Geometry: final body of the model. Coordinates: model frame, mm. Give positions to 0.01 mm unless a question says otherwise; leave off trailing zeros. Write each loop counter-clockwise with the first axis right and the second up, starting at its lowest first coordinate (ties: lowest second). Pieces come first, ordered by that corner, then holes.
Q1. Line query: L1, parallel to X at y = -1.5, z = 0.1; L2, parallel to Y at x = 2.75, z = 0.1; L3, parallel to Y at x = -2, z = 0.15. Output: solid intervals per line, ascending.
Q2. Cut plane D-D on x = 2.5. Return the cut outline in (y, z), plus the area to 3 significant figures.
Q3. Cut plane C-C on y = 2. Return the cut outline in (x, z), plus the area to 3 significant figures.
Q4. Draft query along Y for faces 1 (the face through (1, 0, 0)), 2 (the face through (2.57, -0.62, 0.15)), 3 (the face through (-3.32, 3.04, 0.15)). Return one class per face: pulls with the +Y half, pulls with the -Y half, needs draft (parallel to the pull), parting line crosses it, or undercut.
Q5. Cut plane B-B on y = 0. Return the cut outline in (x, z), plus the area to 3 significant figures.
Q6. Cut plane A-A on x = 0. Return the cut outline in (y, z), plus the area to 3 significant figures.
```python
from build123d import *

# Parameters (mm, degrees)
SKETCH1_R           = 4.5
SKETCH1_R_2         = 0.75
BOSS_EXTRUDE1_DEPTH = 0.3
SKETCH2_R           = 0.25
CUT_EXTRUDE1_DEPTH  = 0.3
SKETCH3_W           = 1.6
SKETCH3_H           = 3
CUT_EXTRUDE2_DEPTH  = 0.3
FILLET1_R           = 0.2
SKETCH4_R           = 0.15
CUT_EXTRUDE3_DEPTH  = 0.3
CIRPATTERN1_COUNT   = 3
SKETCH5_R           = 0.15
CUT_EXTRUDE4_DEPTH  = 0.3
CIRPATTERN3_COUNT   = 3
SKETCH6_R           = 0.15
CUT_EXTRUDE5_DEPTH  = 0.3
CIRPATTERN4_COUNT   = 3
SKETCH7_R           = 0.15
CUT_EXTRUDE8_DEPTH  = 0.3


with BuildPart() as part:
    # Sketch1 → Boss-Extrude1 (new body)
    with BuildSketch(Plane.XY):
        Circle(SKETCH1_R)
        with Locations((0, 2.5)):
            Circle(SKETCH1_R_2, mode=Mode.SUBTRACT)
        with Locations((2.165063509, -1.25)):
            Circle(SKETCH1_R_2, mode=Mode.SUBTRACT)
        with Locations((-2.165063509, -1.25)):
            Circle(SKETCH1_R_2, mode=Mode.SUBTRACT)
    extrude(amount=BOSS_EXTRUDE1_DEPTH)

    # Sketch2 → Cut-Extrude1 (cut)
    with BuildSketch(Plane.XY.offset(0.3)):
        with Locations((0, -4)):
            Circle(SKETCH2_R)
        with Locations((-3.464101615, -2)):
            Circle(SKETCH2_R)
        with Locations((-3.464101615, 2)):
            Circle(SKETCH2_R)
        with Locations((0, 4)):
            Circle(SKETCH2_R)
        with Locations((3.464101615, 2)):
            Circle(SKETCH2_R)
        with Locations((3.464101615, -2)):
            Circle(SKETCH2_R)
    extrude(amount=-CUT_EXTRUDE1_DEPTH, mode=Mode.SUBTRACT)

    # Sketch3 → Cut-Extrude2 (cut)
    with BuildSketch(Plane.XY.offset(0.3)):
        with Locations((0, -1)):
            Rectangle(SKETCH3_W, SKETCH3_H)
    extrude(amount=-CUT_EXTRUDE2_DEPTH, mode=Mode.SUBTRACT)

    # Fillet1
    fillet1_edges = [part.edges().sort_by_distance(p)[0] for p in [
        (-0.8, 0.5, 0.15),
        (0.8, 0.5, 0.15),
        (0.8, -2.5, 0.15),
        (-0.8, -2.5, 0.15),
    ]]
    fillet(fillet1_edges, radius=FILLET1_R)

    # Sketch4 → Cut-Extrude3 (cut)
    with BuildSketch(Plane.XY.offset(0.3)):
        with Locations((0, 3.5)):
            Circle(SKETCH4_R)
    cut_extrude3 = extrude(amount=-CUT_EXTRUDE3_DEPTH, mode=Mode.SUBTRACT)

    # CirPattern1: Cut-Extrude3 ×3 about axis
    cirpattern1_axis = Axis((0, 2.5, 0), (0, 0, 1))
    for i in range(1, CIRPATTERN1_COUNT):
        add(cut_extrude3.rotate(cirpattern1_axis, i * 360 / CIRPATTERN1_COUNT), mode=Mode.SUBTRACT)

    # Sketch5 → Cut-Extrude4 (cut)
    with BuildSketch(Plane.XY.offset(0.3)):
        with Locations((3.165063509, -1.25)):
            Circle(SKETCH5_R)
    cut_extrude4 = extrude(amount=-CUT_EXTRUDE4_DEPTH, mode=Mode.SUBTRACT)

    # CirPattern3: Cut-Extrude4 ×3 about axis
    cirpattern3_axis = Axis((2.165063509, -1.25, 0), (0, 0, 1))
    for i in range(1, CIRPATTERN3_COUNT):
        add(cut_extrude4.rotate(cirpattern3_axis, i * 360 / CIRPATTERN3_COUNT), mode=Mode.SUBTRACT)

    # Sketch6 → Cut-Extrude5 (cut)
    with BuildSketch(Plane.XY.offset(0.3)):
        with Locations((-3.165063509, -1.25)):
            Circle(SKETCH6_R)
    cut_extrude5 = extrude(amount=-CUT_EXTRUDE5_DEPTH, mode=Mode.SUBTRACT)

    # CirPattern4: Cut-Extrude5 ×3 about axis
    cirpattern4_axis = Axis((-2.165063509, -1.25, 0), (0, 0, 1))
    for i in range(1, CIRPATTERN4_COUNT):
        add(cut_extrude5.rotate(cirpattern4_axis, i * 360 / CIRPATTERN4_COUNT), mode=Mode.SUBTRACT)

    # Sketch7 → Cut-Extrude8 (cut)
    with BuildSketch(Plane.XY.offset(0.3)):
        with Locations((0.4, -3)):
            Circle(SKETCH7_R)
        with Locations((-0.4, -3)):
            Circle(SKETCH7_R)
        with Locations((0.4, 1)):
            Circle(SKETCH7_R)
        with Locations((-0.4, 1)):
            Circle(SKETCH7_R)
    extrude(amount=-CUT_EXTRUDE8_DEPTH, mode=Mode.SUBTRACT)


solid = part.part
```
Data:
1. L1: x = -4.24 to -2.87, -1.46 to -0.8, 0.8 to 1.46, 2.87 to 4.24
1. L2: y = -3.56 to -1.72, -0.78 to 3.56
1. L3: y = -4.03 to -1.98, -0.52 to 4.03
2. outline: (-3.74, 0) - (-1.92, 0) - (-1.92, 0.3) - (-3.74, 0.3) - close; (-0.58, 0) - (3.74, 0) - (3.74, 0.3) - (-0.58, 0.3) - close
2. area: 1.84 mm2
3. outline: (-4.03, 0) - (-3.71, 0) - (-3.71, 0.3) - (-4.03, 0.3) - close; (-3.21, 0) - (-1.02, 0) - (-1.02, 0.3) - (-3.21, 0.3) - close; (-0.72, 0) - (-0.56, 0) - (-0.56, 0.3) - (-0.72, 0.3) - close; (0.56, 0) - (0.72, 0) - (0.72, 0.3) - (0.56, 0.3) - close; (1.02, 0) - (3.21, 0) - (3.21, 0.3) - (1.02, 0.3) - close; (3.71, 0) - (4.03, 0) - (4.03, 0.3) - (3.71, 0.3) - close
3. area: 1.60 mm2
4. face 1: needs draft
4. face 2: undercut
4. face 3: parting line crosses it
5. outline: (-4.5, 0) - (-0.8, 0) - (-0.8, 0.3) - (-4.5, 0.3) - close; (0.8, 0) - (4.5, 0) - (4.5, 0.3) - (0.8, 0.3) - close
5. area: 2.22 mm2
6. outline: (-4.5, 0) - (-4.25, 0) - (-4.25, 0.3) - (-4.5, 0.3) - close; (-3.75, 0) - (-2.5, 0) - (-2.5, 0.3) - (-3.75, 0.3) - close; (0.5, 0) - (1.75, 0) - (1.75, 0.3) - (0.5, 0.3) - close; (3.25, 0) - (3.35, 0) - (3.35, 0.3) - (3.25, 0.3) - close; (3.65, 0) - (3.75, 0) - (3.75, 0.3) - (3.65, 0.3) - close; (4.25, 0) - (4.5, 0) - (4.5, 0.3) - (4.25, 0.3) - close
6. area: 0.960 mm2
